Can you work these out from the model? Positions are in its coordinate system, mm. A direction names the side the tool comes from. Give positions to 0.01 mm unless a question says otherwise; leave off trailing zeros. Loops run counter-clockwise (first coordinate to the right, second up) from the corner with the lowest first, then second, coordinate; pieces in that order, holes last. Notation, with made-up numbers: (64.25, -33.75) -> (83.25, -33.75) arc R19 cw to (83.25, -7.75) -> close; hole circle Ø6 at (47.25, 37.5). An arc over 180 degrees is marked (long way). Return JSON: item names as keys, results as strings. Group by question number.
Q1. Suppose I cut it at D-D, the plane z = 26. Please give me the cut outline in (x, y), and give its area (3 significant figures).
Q2. I need wall thicknesses on line 1 along Z through (x, y) = (-8.5, 14.5); line 2 along Y through (x, z) = (0, 22.5); line 3 along Z through (x, y) = (-0.5, -13). Which ranges of each line are inside material? Lowest first, please. Write a range as [from, to].
Q3. Suppose I cut it at A-A, the plane y = 16. Please give me the cut outline in (x, z), and give its area (3 significant figures).
Q4. Which directions (+Z, -Z, +X, -X, +Y, -Y) give clear straight access to the entire face, cutting with the end or side of a thin tool? Please do faces 1 (the flat face through (0, 21.924, 29)), 2 (the flat face through (0, 24.557, 30)), 3 (the flat face through (0, 23, 22.265)), 4 (the flat face through (0, 14, 29.112)).
Q5. Thinking about a two-plate mould opening in X: for faces 5 (the flat face through (0, 16, 30.799)), 6 (the flat face through (-19.587, 6, 7)), 7 (the flat face through (-16.846, 15, 22)), 8 (the flat face through (0, 17, 37.633)), which applies, pulls with the +X half, pulls with the -X half, needs draft (parallel to the pull), parting line crosses it, or undercut?
Q6. Suppose I cut it at B-B, the plane z = 36. Please give me the cut outline in (x, y).
Q7. Suppose I cut it at C-C, the plane x = -12. Please give me the cut outline in (y, z).
Q8. Will these pins go through, and if not, where does the flat tip stop? pin 1 (6 mm diameter, centred on x = -15, y = -5, fed in from +Z); pin 2 (3 mm diameter, centred on x = 1.5, z = 37.5, fed in from +Y); pin 3 (22 mm diameter, centred on x = 5.5, z = 24.5, fed in from -Y).
```python
from build123d import *

# Parameters (mm, degrees)
F0_W     = 2.7405302972
F0_H     = 12.7354152501
F1_DEPTH = 10
F2_DEPTH = 35
F3_R     = 1.6440039884
F4_DEPTH = 33.6924307048
F6_DEPTH = 39.1734912992
F8_DEPTH = 5


with BuildPart() as f1:
    # F0 (on Top) → F1 (new body)
    with BuildSketch(Plane.XY):
        Polygon((19.5867456496, 29.3398164213), (-19.5867456496, 29.3398164213), (-19.5867456496, 21.9242591411), (-16.8462153524, 21.9242591411), (-16.8462153524, 9.188843891), (-19.5867456496, 9.188843891), (-19.5867456496, -29.3398164213), (19.5867456496, -29.3398164213), (19.5867456496, 9.188843891), (16.8462153524, 9.188843891), (16.8462153524, 21.9242591411), (19.5867456496, 21.9242591411), align=None)
        with Locations((-18.216480501, 15.5565515161)):
            Rectangle(F0_W, F0_H)
        with Locations((18.216480501, 15.5565515161)):
            Rectangle(F0_W, F0_H)
    extrude(amount=F1_DEPTH)

    # F0 (on Top) → F2 (join)
    with BuildSketch(Plane.XY):
        with Locations((-18.216480501, 15.5565515161)):
            Rectangle(F0_W, F0_H)
        with Locations((18.216480501, 15.5565515161)):
            Rectangle(F0_W, F0_H)
    extrude(amount=F2_DEPTH)

    # F3 (on face) → F4 (join, through all)
    with BuildSketch(Plane.YZ.offset(-16.8462153524)):
        with Locations((12.3588815841, 32.1788525892)):
            Circle(F3_R)
        with Locations((18.754221448, 32.1788525892)):
            Circle(F3_R)
    extrude(amount=F4_DEPTH)

    # F5 (on face) → F6 (join, through all)
    with BuildSketch(Plane.YZ.offset(19.5867456496)):
        Polygon((9.188843891, 37.6330949366), (9.188843891, 35), (21.9242591411, 35), (21.9242591411, 22.2645847499), (24.5573540777, 22.2645847499), (24.5573540777, 37.6330949366), align=None)
    extrude(amount=-F6_DEPTH)

    # F7 (on Right) → F8 (join, symmetric)
    with BuildSketch(Plane.YZ):
        Polygon((19.9882956222, 29.1119106114), (19.9882956222, 30.7994605973), (9.100439027, 30.7994605973), (9.100439027, 41.6873171926), (7.412889041, 41.6873171926), (7.412889041, 29.1119106114), align=None)
    extrude(amount=F8_DEPTH, both=True)


solid = f1.part
```
Ans:
{
 "1": {"outline": "(-19.59, 9.19) -> (-16.85, 9.19) -> (-16.85, 21.92) -> (16.85, 21.92) -> (16.85, 9.19) -> (19.59, 9.19) -> (19.59, 24.56) -> (-19.59, 24.56) -> close", "area": "173 mm^2"},
 "2": {"line 1": "z = [0, 10], [35, 37.63]", "line 2": "y = [21.92, 24.56]", "line 3": "z = [0, 10]"},
 "3": {"outline": "(-19.59, 0) -> (19.59, 0) -> (19.59, 37.63) -> (-19.59, 37.63) -> close; (-5, 29.11) -> (5, 29.11) -> (5, 30.8) -> (-5, 30.8) -> close; hole (-16.85, 10) -> (16.85, 10) -> (16.85, 35) -> (-16.85, 35) -> close", "area": "649 mm^2"},
 "4": {"face 1": "none", "face 2": "+Z, +X, -X, +Y", "face 3": "+X, -X, +Y", "face 4": "-Y"},
 "5": {"face 5": "undercut", "face 6": "pulls with the -X half", "face 7": "undercut", "face 8": "needs draft"},
 "6": {"outline": "(-19.59, 9.19) -> (19.59, 9.19) -> (19.59, 24.56) -> (-19.59, 24.56) -> close; (-5, 7.41) -> (5, 7.41) -> (5, 9.1) -> (-5, 9.1) -> close"},
 "7": {"outline": "(-29.34, 0) -> (29.34, 0) -> (29.34, 10) -> (-29.34, 10) -> close; (9.19, 35) -> (21.92, 35) -> (21.92, 22.26) -> (24.56, 22.26) -> (24.56, 37.63) -> (9.19, 37.63) -> close; circle Ø3.29 at (12.36, 32.18); circle Ø3.29 at (18.75, 32.18)"},
 "8": {"pin 1": "stops at z = 10", "pin 2": "stops at y = 24.56", "pin 3": "stops at y = 7.41"}
}
